from build123d import *

# Parameters (mm, degrees)
F1_DEPTH = 22.86
F3_DEPTH = 21.59
F4_R     = 5.7920726269
F4_R_2   = 5.6767618258
F5_DEPTH = 25.4
F6_W     = 15.9551920369
F6_H     = 6.0370992869
F6_W_2   = 15.0927454233
F6_H_2   = 6.4683184028
F7_DEPTH = 12.9
F8_DEPTH = 16.1
F9_DEPTH = 30.8


with BuildPart() as f1:
    # F0 (on Front) → F1 (new body)
    with BuildSketch(Plane.XZ):
        with BuildLine():
            ThreePointArc((-50.7977157831, -20.9915483534), (-48.9378438437, -25.481676414), (-44.4477157831, -27.3415483534))
            Line((-44.4477157831, -27.3415483534), (44.4477157831, -27.3415483534))
            ThreePointArc((44.4477157831, -27.3415483534), (48.9378438437, -25.481676414), (50.7977157831, -20.9915483534))
            Line((50.7977157831, -20.9915483534), (50.7977157831, 20.9915483534))
            ThreePointArc((50.7977157831, 20.9915483534), (48.9378438437, 25.481676414), (44.4477157831, 27.3415483534))
            Line((44.4477157831, 27.3415483534), (-44.4477157831, 27.3415483534))
            ThreePointArc((-44.4477157831, 27.3415483534), (-48.9378438437, 25.481676414), (-50.7977157831, 20.9915483534))
            Line((-50.7977157831, 20.9915483534), (-50.7977157831, -20.9915483534))
        make_face()
        with BuildLine():
            Line((37.8281841218, -17.8439579904), (-37.8281841218, -17.8439579904))
            ThreePointArc((-37.8281841218, -17.8439579904), (-42.3183121824, -15.9840860509), (-44.1781841218, -11.4939579904))
            Line((-44.1781841218, -11.4939579904), (-44.1781841218, 11.4939579904))
            ThreePointArc((-44.1781841218, 11.4939579904), (-42.3183121824, 15.9840860509), (-37.8281841218, 17.8439579904))
            Line((-37.8281841218, 17.8439579904), (37.8281841218, 17.8439579904))
            ThreePointArc((37.8281841218, 17.8439579904), (42.3183121824, 15.9840860509), (44.1781841218, 11.4939579904))
            Line((44.1781841218, 11.4939579904), (44.1781841218, -11.4939579904))
            ThreePointArc((44.1781841218, -11.4939579904), (42.3183121824, -15.9840860509), (37.8281841218, -17.8439579904))
        make_face(mode=Mode.SUBTRACT)
        with BuildLine():
            ThreePointArc((-44.1781841218, -11.4939579904), (-42.3183121824, -15.9840860509), (-37.8281841218, -17.8439579904))
            Line((-37.8281841218, -17.8439579904), (37.8281841218, -17.8439579904))
            ThreePointArc((37.8281841218, -17.8439579904), (42.3183121824, -15.9840860509), (44.1781841218, -11.4939579904))
            Line((44.1781841218, -11.4939579904), (44.1781841218, 11.4939579904))
            ThreePointArc((44.1781841218, 11.4939579904), (42.3183121824, 15.9840860509), (37.8281841218, 17.8439579904))
            Line((37.8281841218, 17.8439579904), (-37.8281841218, 17.8439579904))
            ThreePointArc((-37.8281841218, 17.8439579904), (-42.3183121824, 15.9840860509), (-44.1781841218, 11.4939579904))
            Line((-44.1781841218, 11.4939579904), (-44.1781841218, -11.4939579904))
        make_face()
    extrude(amount=-F1_DEPTH)

    # F2 (on Front) → F3 (cut)
    with BuildSketch(Plane.XZ):
        with BuildLine():
            Line((-41.7135613203, -22.448848933), (41.7135613203, -22.448848933))
            ThreePointArc((41.7135613203, -22.448848933), (46.2036893808, -20.5889769935), (48.0635613203, -16.098848933))
            Line((48.0635613203, -16.098848933), (48.0635613203, 16.098848933))
            ThreePointArc((48.0635613203, 16.098848933), (46.2036893808, 20.5889769935), (41.7135613203, 22.448848933))
            Line((41.7135613203, 22.448848933), (-41.7135613203, 22.448848933))
            ThreePointArc((-41.7135613203, 22.448848933), (-46.2036893808, 20.5889769935), (-48.0635613203, 16.098848933))
            Line((-48.0635613203, 16.098848933), (-48.0635613203, -16.098848933))
            ThreePointArc((-48.0635613203, -16.098848933), (-46.2036893808, -20.5889769935), (-41.7135613203, -22.448848933))
        make_face()
    extrude(amount=-F3_DEPTH, mode=Mode.SUBTRACT)

    # F4 (on face) → F5 (cut)
    with BuildSketch(Plane.XZ.offset(-21.59)):
        with Locations((-38.1261706352, 12.0878387243)):
            Circle(F4_R)
        with Locations((-1.2961706352, 12.0878387243)):
            Circle(F4_R)
        with Locations((35.5338293648, 12.0878387243)):
            Circle(F4_R)
        with Locations((-38.9896593988, -12.66345568)):
            Circle(F4_R_2)
        with Locations((-0.8896593988, -12.66345568)):
            Circle(F4_R_2)
        with Locations((37.2103406012, -12.66345568)):
            Circle(F4_R_2)
    extrude(amount=-F5_DEPTH, mode=Mode.SUBTRACT)

    # F6 (on face) → F7 (join)
    with BuildSketch(Plane(origin=(0, 22.86, 0), x_dir=(-1, 0, 0), z_dir=(0, 1, 0))):
        with Locations((-20.4493920319, 20.0157957152)):
            Rectangle(F6_W, F6_H)
        with Locations((20.9506079681, 20.0157957152)):
            Rectangle(F6_W, F6_H)
        with Locations((-19.3713400513, -20.7346286625)):
            Rectangle(F6_W_2, F6_H_2)
        with Locations((24.1286599487, -20.7346286625)):
            Rectangle(F6_W_2, F6_H_2)
    extrude(amount=F7_DEPTH)

    # F8 (cut): a face of the model
    f8_faces = [f1.faces().sort_by_distance(p)[0] for p in [
        (-48.1220046199, 0, 24.6658371902),
    ]]
    extrude(f8_faces, amount=-F8_DEPTH, mode=Mode.SUBTRACT)

    # F9 (add): faces of the model
    f9_faces = [f1.faces().sort_by_distance(p)[0] for p in [
        (20.4493920319, 35.76, 20.0157957152),
        (-20.9506079681, 35.76, 20.0157957152),
        (-24.1286599487, 35.76, -20.7346286625),
        (19.3713400513, 35.76, -20.7346286625),
    ]]
    extrude(f9_faces, amount=-F9_DEPTH)


solid = f1.part
Design review of the part built by this model. Coordinates are the model's own, in mm. A direction names the side the tool comes from. Round coordinates to 2 decimals unless told otherwise and drop trailing zeros. Write each loop counter-clockwise with the first axis right and the second up, starting at its lowest first coordinate (ties: lowest second). Pieces come first, ordered by that corner, then holes. Notation, with made-up numbers: (-34, 0.25) - (-7, 0.25) arc R6 ccw to (-7, 6.25) - close; hole circle Ø7 at (-14, 2). An arc over 180 degrees is marked (long way). Return JSON: item names as keys, results as strings. Group by question number.
Item 1: For probe 1 along X at (y, z) = (7, 23); probe 2 along Z at (x, y) = (7, 20); probe 3 along X at (y, z) = (16.5, -7.5), list the stretches that pass through material, from the lowest coordinate up. Write a range as [from, to].
Item 2: Insertion check: P1, Ø1.8, axis at y = 12, z = 21, coming from the -X side; P2, Ø3.5, axis at x = 17, y = 8.5, coming from the -Z side; P3, Ø15, axis at x = 37.21, z = -12.66, coming from the +Y side; P4, Ø6, axis at x = 0.5, z = -10.5, coming from the +Y side. Each pin has a flat end and moves straight along its axis. Give the tip position at first contact, or say it passes through.
Item 3: We need section C-C on y = 28. Write out the cut boundary in (x, z), and give its area (3 significant figures).
Item 4: We need section D-D on z = 7.5. Write out the cut boundary in (x, y), and give its area (3 significant figures).
Item 5: We need section B-B on x = 8. Write out the cut boundary in (y, z), and give its area (3 significant figures).
Item 6: Machinability: for faces 4 (the face through (-48.064, 19, 0)), 5 (the face through (19, 29, -23.969)), 6 (the face through (-21, 11, 23.034)), which of the approach directions +Z, -Z, +X, -X, +Y, -Y give a long, thin tool a straight path to every point of the face, cutting with its end or side? Answer none if there is none.
Item 7: The part is to be moulded in two halves that separate along Z. For faces 1 (the face through (-24, 29, -17.5)), 2 (the face through (-21, 35.76, 20)), 3 (the face through (48.99, 19.43, 25.43)), say which applies: pulls with the +Z half, pulls with the -Z half, needs draft (parallel to the pull), parting line crosses it, or undercut.
Model answer:
{
 "1": {"probe 1": "x = [-28.93, -12.97], [12.47, 28.43]", "probe 2": "z = [-27.34, -22.45], [22.45, 27.34]", "probe 3": "x = [-50.8, -48.06], [48.06, 50.8]"},
 "2": {"P1": "stops at x = -28.93", "P2": "stops at z = -23.97", "P3": "stops at y = 22.86", "P4": "passes through"},
 "3": {"outline": "(-31.68, -23.97) - (-16.58, -23.97) - (-16.58, -17.5) - (-31.68, -17.5) - close; (-28.93, 17) - (-12.97, 17) - (-12.97, 23.03) - (-28.93, 23.03) - close; (11.82, -23.97) - (26.92, -23.97) - (26.92, -17.5) - (11.82, -17.5) - close; (12.47, 17) - (28.43, 17) - (28.43, 23.03) - (12.47, 23.03) - close", "area": "388 mm²"},
 "4": {"outline": "(-50.8, 16.1) - (-48.06, 16.1) - (-48.06, 21.59) - (-41.66, 21.59) - (-41.66, 22.86) - (-50.8, 22.86) - close; (-34.59, 21.59) - (-4.83, 21.59) - (-4.83, 22.86) - (-34.59, 22.86) - close; (2.24, 21.59) - (32, 21.59) - (32, 22.86) - (2.24, 22.86) - close; (39.07, 21.59) - (48.06, 21.59) - (48.06, 16.1) - (50.8, 16.1) - (50.8, 22.86) - (39.07, 22.86) - close", "area": "132 mm²"},
 "5": {"outline": "(16.1, -27.34) - (22.86, -27.34) - (22.86, 27.34) - (16.1, 27.34) - (16.1, 22.45) - (21.59, 22.45) - (21.59, -22.45) - (16.1, -22.45) - close", "area": "123 mm²"},
 "6": {"face 4": "-Y", "face 5": "-Z, +X, -X, +Y", "face 6": "+Z, +X, -X, -Y"},
 "7": {"face 1": "undercut", "face 2": "needs draft", "face 3": "pulls with the +Z half"}
}
